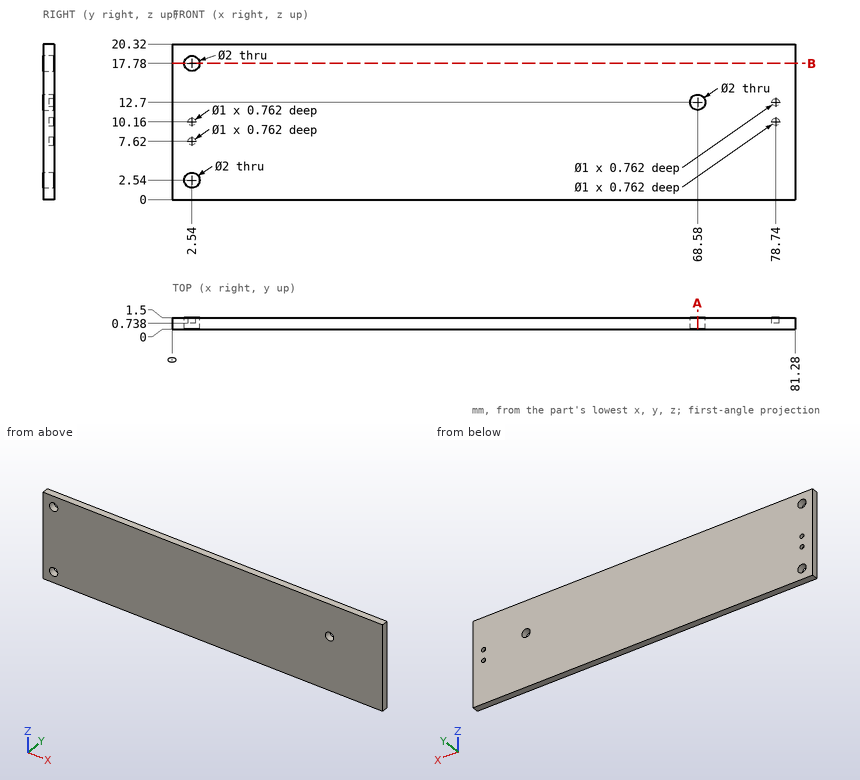
Geometry check sheet. Reference: drawing and pictorial views, mm from the part's lowest x, y, z. Coordinates: 2 decimals unless noted, no trailing zeros. Order: outer loops, then holes, each group sorted by start corner. A loop starts at its lowest first (then second) coordinate and runs counter-clockwise, first axis right, second up.
1. Sectioned sample at B-B, the plane z = 17.78. Record the cut outline in (x, y).
Results found:
outline: (0, 0) - (1.54, 0) - (1.54, 1.5) - (0, 1.5) - close; (3.54, 0) - (81.28, 0) - (81.28, 1.5) - (3.54, 1.5) - close
2. Sectioned sample at A-A, the plane x = 68.58. Record the cut outline in (y, z).
Results found:
outline: (0, 0) - (1.5, 0) - (1.5, 11.7) - (0, 11.7) - close; (0, 13.7) - (1.5, 13.7) - (1.5, 20.32) - (0, 20.32) - close
3. Go/stop test with a flat-tipped pin: pin 1 Ø1.2 at (x, z) = (68.58, 12.7) entering from -Y. Record where the tip stops, or that it passes through.
Results found:
pin 1: passes through
4. Scan lines: line 1 (X direction, y = 1.1, z = 10.16); line 2 (Z direction, x = 78.74, y = 1.3); line 3 (X direction, y = 0.55, z = 17.78). Record each from-to range of solid material in increasing order.
Results found:
line 1: x = 0 to 2.04, 3.04 to 78.24, 79.24 to 81.28
line 2: z = 0 to 9.66, 10.66 to 12.2, 13.2 to 20.32
line 3: x = 0 to 1.54, 3.54 to 81.28
